The listing builds one solid part. Answer for the finished solid, in the listing's coordinates (mm). Face numbers are marked on the shaded views. A direction names the side the tool comes from. Coordinates: 2 decimals unless noted, no trailing zeros. Loops run counter-clockwise (first coordinate to the right, second up) from the corner with the lowest first, then second, coordinate; pieces in that order, holes last. Notation, with made-up numbers: M -22.5,34.25 L 5.5,34.25 A26 cw 5.5,64.25 Z; hole C 65,68.5 d4. An arc over 180 degrees is marked long. Answer in a Markdown table with one row per item. Add a question column.
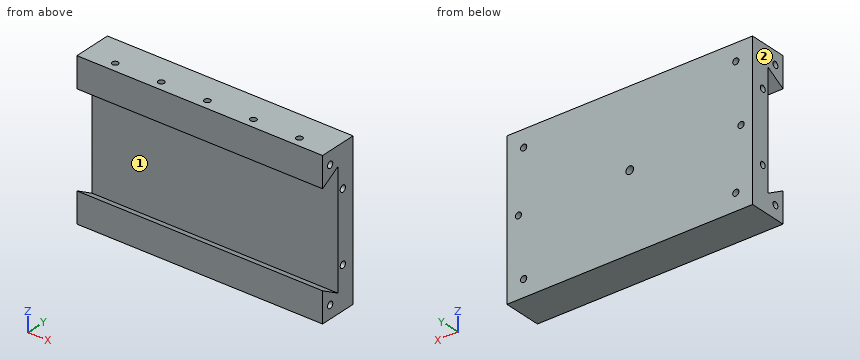
from build123d import *

# Parameters (mm, degrees)
FEMALE_DOVETAIL_EXTRUDE_DEPTH                = 203.2
END_PLATES_1_4_28_TAPPED_HOLE_D              = 5.1054
END_PLATES_1_4_28_TAPPED_HOLE_DEPTH          = 16.51
END_PLATES_1_4_28_TAPPED_HOLE_TIP            = 1.533816902
END_PLATES_1_4_28_TAPPED_HOLE1_D             = 5.4102
END_PLATES_1_4_28_TAPPED_HOLE1_DEPTH         = 15.494
END_PLATES_1_4_28_TAPPED_HOLE1_TIP           = 1.625388061
SWIVEL_BLOCK_MOUNT_1_4_20_TAPPED_HOLE5_D     = 5.1054
SWIVEL_BLOCK_MOUNT_1_4_20_TAPPED_HOLE5_DEPTH = 10.16
SWIVEL_BLOCK_MOUNT_1_4_20_TAPPED_HOLE5_TIP   = 1.533816902
SWIVEL_LOCATING_1_4_0_25_CLEARANCE_DOW_D     = 6.35
SWIVEL_LOCATING_1_4_0_25_CLEARANCE_DOW_DEPTH = 6.35
SKETCH22_W                                   = 2.5527
SKETCH22_H                                   = 63.5
GIB_SCREW_1_4_20_TAPPED_HOLE6_AT_2_COUNT     = 2
GIB_SCREW_1_4_20_TAPPED_HOLE6_AT_2_PITCH     = 38.1
GIB_SCREW_1_4_20_TAPPED_HOLE6_AT_3_COUNT     = 2
GIB_SCREW_1_4_20_TAPPED_HOLE6_AT_3_PITCH     = 76.2
GIB_SCREW_1_4_20_TAPPED_HOLE6_AT_4_COUNT     = 2
GIB_SCREW_1_4_20_TAPPED_HOLE6_AT_4_PITCH     = 114.3
GIB_SCREW_1_4_20_TAPPED_HOLE6_AT_5_COUNT     = 2
GIB_SCREW_1_4_20_TAPPED_HOLE6_AT_5_PITCH     = 152.4


with BuildPart() as part:
    # Sketch1 → female dovetail extrude (new body)
    with BuildSketch(Plane(origin=(0, 0, 0), x_dir=(0, 0, -1), z_dir=(1, 0, 0))):
        Polygon((63.5, 31.75), (-63.5, 31.75), (-63.5, 0), (-38.459564477, 0), (-47.625, 15.875), (-40.292651581, 15.875), (-16.056336319, 15.875), (16.056336319, 15.875), (47.625, 15.875), (38.459564477, 0), (63.5, 0), align=None)
    extrude(amount=FEMALE_DOVETAIL_EXTRUDE_DEPTH)

    # end plates 1/4-28 Tapped Hole
    with Locations(Plane(origin=(0, -44.45, -248.332419753), x_dir=(0, 0, 1), z_dir=(-1, 0, 0))):
        with Locations((195.500419753, 52.3875), (219.630419753, 65.532), (277.034419753, 65.532), (301.164419753, 52.3875)):
            Hole(END_PLATES_1_4_28_TAPPED_HOLE_D / 2, depth=END_PLATES_1_4_28_TAPPED_HOLE_DEPTH)
            with Locations((0, 0, -(END_PLATES_1_4_28_TAPPED_HOLE_DEPTH + END_PLATES_1_4_28_TAPPED_HOLE_TIP / 2))):  # 118° drill point
                Cone(0, END_PLATES_1_4_28_TAPPED_HOLE_D / 2, END_PLATES_1_4_28_TAPPED_HOLE_TIP, mode=Mode.SUBTRACT)

    # end plates 1/4-28 Tapped Hole1
    with Locations(Plane(origin=(203.2, -44.45, -248.332419753), x_dir=(0, 0, -1), z_dir=(1, 0, 0))):
        with Locations((-301.164419753, 52.3875), (-277.034419753, 65.532), (-219.630419753, 65.532), (-195.500419753, 52.3875)):
            Hole(END_PLATES_1_4_28_TAPPED_HOLE1_D / 2, depth=END_PLATES_1_4_28_TAPPED_HOLE1_DEPTH)
            with Locations((0, 0, -(END_PLATES_1_4_28_TAPPED_HOLE1_DEPTH + END_PLATES_1_4_28_TAPPED_HOLE1_TIP / 2))):  # 118° drill point
                Cone(0, END_PLATES_1_4_28_TAPPED_HOLE1_D / 2, END_PLATES_1_4_28_TAPPED_HOLE1_TIP, mode=Mode.SUBTRACT)

    # swivel block mount 1/4-20 Tapped Hole5
    with Locations(Plane(origin=(0, 31.75, 0), x_dir=(1, 0, 0), z_dir=(0, 1, 0))):
        with Locations((13.843, -49.53), (9.525, 0), (13.843, 49.53), (189.357, 49.53), (193.675, 0), (189.357, -49.53)):
            Hole(SWIVEL_BLOCK_MOUNT_1_4_20_TAPPED_HOLE5_D / 2, depth=SWIVEL_BLOCK_MOUNT_1_4_20_TAPPED_HOLE5_DEPTH)
            with Locations((0, 0, -(SWIVEL_BLOCK_MOUNT_1_4_20_TAPPED_HOLE5_DEPTH + SWIVEL_BLOCK_MOUNT_1_4_20_TAPPED_HOLE5_TIP / 2))):  # 118° drill point
                Cone(0, SWIVEL_BLOCK_MOUNT_1_4_20_TAPPED_HOLE5_D / 2, SWIVEL_BLOCK_MOUNT_1_4_20_TAPPED_HOLE5_TIP, mode=Mode.SUBTRACT)

    # swivel locating 1/4 (0.25) Clearance Dowel Hole1
    with Locations(Plane(origin=(39.932785273, 31.75, 145.909625699), x_dir=(1, 0, 0), z_dir=(0, 1, 0))):
        with Locations((61.667214727, 145.909625699)):
            Hole(SWIVEL_LOCATING_1_4_0_25_CLEARANCE_DOW_D / 2, depth=SWIVEL_LOCATING_1_4_0_25_CLEARANCE_DOW_DEPTH)

    # Sketch22 → gib screw 1/4-20 Tapped Hole6 (revolve, cut)
    with BuildSketch(Plane(origin=(25.4, 7.9375, 0), x_dir=(0, 1, 0), z_dir=(1, 0, 0))):
        with Locations((1.27635, 31.75)):
            Rectangle(SKETCH22_W, SKETCH22_H)
    gib_screw_1_4_20_tapped_hole6 = revolve(axis=Axis((25.4, 7.9375, -6.35), (0, 0, 1)), mode=Mode.SUBTRACT)

    # gib screw 1/4-20 Tapped Hole6 at 2: gib screw 1/4-20 Tapped Hole6 ×2
    with Locations(*[(i * GIB_SCREW_1_4_20_TAPPED_HOLE6_AT_2_PITCH, 0, 0) for i in range(1, GIB_SCREW_1_4_20_TAPPED_HOLE6_AT_2_COUNT)]):
        add(gib_screw_1_4_20_tapped_hole6, mode=Mode.SUBTRACT)

    # gib screw 1/4-20 Tapped Hole6 at 3: gib screw 1/4-20 Tapped Hole6 ×2
    with Locations(*[(i * GIB_SCREW_1_4_20_TAPPED_HOLE6_AT_3_PITCH, 0, 0) for i in range(1, GIB_SCREW_1_4_20_TAPPED_HOLE6_AT_3_COUNT)]):
        add(gib_screw_1_4_20_tapped_hole6, mode=Mode.SUBTRACT)

    # gib screw 1/4-20 Tapped Hole6 at 4: gib screw 1/4-20 Tapped Hole6 ×2
    with Locations(*[(i * GIB_SCREW_1_4_20_TAPPED_HOLE6_AT_4_PITCH, 0, 0) for i in range(1, GIB_SCREW_1_4_20_TAPPED_HOLE6_AT_4_COUNT)]):
        add(gib_screw_1_4_20_tapped_hole6, mode=Mode.SUBTRACT)

    # gib screw 1/4-20 Tapped Hole6 at 5: gib screw 1/4-20 Tapped Hole6 ×2
    with Locations(*[(i * GIB_SCREW_1_4_20_TAPPED_HOLE6_AT_5_PITCH, 0, 0) for i in range(1, GIB_SCREW_1_4_20_TAPPED_HOLE6_AT_5_COUNT)]):
        add(gib_screw_1_4_20_tapped_hole6, mode=Mode.SUBTRACT)


solid = part.part
(1) Straight lines are drawn through the part: line 1 (X direction, y = 23, z = -49.5); line 2 (Y direction, x = 97, z = 23.5) (3 decimals); line 3 (Y direction, x = 139.7, z = 55.75). For each, find the intervals that lie inside material, in ascending order.
(2) Each of these flat-tipped pins is pushed along its axis until it touches: pin 1 (6.5 mm diameter, centred on x = 13.843, z = 49.53, fed in from +Y); pin 2 (3 mm diameter, centred on x = 64.5, z = -1.5, fed in from -Y) (3 decimals); pin 3 (3 mm diameter, centred on y = 21.082, z = -28.702, fed in from +X); pin 4 (1.9 mm diameter, centred on x = 102, z = -1.5, fed in from +Y). Where does it stop, or does it pass through?
(3) A cutting plane is placed at C-C (x = 101.6). Give the vertices of the cut face in (y, z) (3 decimals).
(4) A cutting plane is placed at A-A (x = 177.8). Give the vertices of the cut face in (y, z) (3 decimals), plus the area to 3 significant figures.
(5) For the marked faces 1 and 2, determine the directions among +Z, -Z, +X, -X, +Y, -Y from which every point of the face is accessible in a straight line to the end or side of a thin tool.
(6) A cutting plane is placed at B-B (z = -41.5). Give the vertices of the cut face in (x, y) (3 decimals).
Solved:
| question | item | result |
|---|---|---|
| 1 | line 1 | x = 0 to 11.29, 16.4 to 186.8, 191.91 to 203.2 |
| 1 | line 2 | y = 15.875 to 31.75 |
| 1 | line 3 | y = 0 to 5.38, 10.49 to 31.75 |
| 2 | pin 1 | stops at y = 31.75 |
| 2 | pin 2 | stops at y = 15.875 |
| 2 | pin 3 | stops at x = 186.98 |
| 2 | pin 4 | stops at y = 25.4 |
| 3 | outline | M 0,-63.5 L 31.75,-63.5 L 31.75,-3.175 L 25.4,-3.175 L 25.4,3.175 L 31.75,3.175 L 31.75,63.5 L 10.49,63.5 L 10.49,44.516 L 15.875,47.625 L 15.875,-47.625 L 0,-38.46 Z; M 0,38.46 L 5.385,41.568 L 5.385,63.5 L 0,63.5 Z |
| 4 | outline | M 0,-63.5 L 31.75,-63.5 L 31.75,63.5 L 10.49,63.5 L 10.49,44.516 L 15.875,47.625 L 15.875,-47.625 L 0,-38.46 Z; M 0,38.46 L 5.385,41.568 L 5.385,63.5 L 0,63.5 Z |
| 4 | area | 2,560 mm² |
| 5 | face 1 | +X, -X |
| 5 | face 2 | +Z, -Z, -X, +Y, -Y |
| 6 | outline | M 0,0 L 203.2,0 L 203.2,5.266 L 0,5.266 Z; M 0,15.875 L 203.2,15.875 L 203.2,31.75 L 0,31.75 Z |
